Check sheet for the modelled part. Datum: model origin and axes. Units: mm. A direction names the side the tool comes from. Round coordinates to 2 decimals unless told otherwise and drop trailing zeros. Write each loop counter-clockwise with the first axis right and the second up, starting at its lowest first coordinate (ties: lowest second). Pieces come first, ordered by that corner, then holes. Notation, with made-up numbers: (-20.5, 78) -> (-9.5, 78) arc R14 ccw to (-9.5, 95) -> close; hole circle Ø10 at (81, 33). An arc over 180 degrees is marked (long way). One line per item, written item: value.
from build123d import *

# Parameters (mm, degrees)
SKETCH_W     = 40
SKETCH_H     = 7
SKETCH_R     = 1.6
PAD_DEPTH    = 7.25
POCKET_DEPTH = 3
FILLET_R     = 3


with BuildPart() as part:
    # Sketch → Pad (new body)
    with BuildSketch(Plane.XY):
        Rectangle(SKETCH_W, SKETCH_H)
        with Locations((-14.85, 0)):
            Circle(SKETCH_R, mode=Mode.SUBTRACT)
        with Locations((14.85, 0)):
            Circle(SKETCH_R, mode=Mode.SUBTRACT)
    extrude(amount=PAD_DEPTH)

    # Sketch001 (on Face8 of Pad) → Pocket (cut)
    with BuildSketch(Plane.XY.offset(7.25)):
        Polygon((-11.616838, 0), (-13.233419, 2.8), (-16.466581, 2.8), (-18.083162, 0), (-16.466581, -2.8), (-13.233419, -2.8), align=None)
        Polygon((11.616838, 0), (13.233419, -2.8), (16.466581, -2.8), (18.083162, 0), (16.466581, 2.8), (13.233419, 2.8), align=None)
    extrude(amount=-POCKET_DEPTH, mode=Mode.SUBTRACT)

    # Fillet
    fillet_edges = [part.edges().sort_by_distance(p)[0] for p in [
        (20, -3.5, 3.625),
        (20, 3.5, 3.625),
        (-20, 3.5, 3.625),
        (-20, -3.5, 3.625),
    ]]
    fillet(fillet_edges, radius=FILLET_R)


solid = part.part
Item 1: Sectioned sample at D-D (z = 6). Enter the section's corners in (x, y), then the cut area to 3 significant figures.
Result set:
outline: (-20, -0.5) arc R3 ccw to (-17, -3.5) -> (17, -3.5) arc R3 ccw to (20, -0.5) -> (20, 0.5) arc R3 ccw to (17, 3.5) -> (-17, 3.5) arc R3 ccw to (-20, 0.5) -> close; hole (-18.08, 0) -> (-16.47, -2.8) -> (-13.23, -2.8) -> (-11.62, 0) -> (-13.23, 2.8) -> (-16.47, 2.8) -> close; hole (11.62, 0) -> (13.23, -2.8) -> (16.47, -2.8) -> (18.08, 0) -> (16.47, 2.8) -> (13.23, 2.8) -> close
area: 218 mm^2
Item 2: Depth check by flat-ended pin: pin 1 (3.5 mm diameter, centred on x = 14.85, y = 0, fed in from +Z); pin 2 (1 mm diameter, centred on x = -5, y = -1.5, fed in from -Z). Enter the tip coordinate at first touch or a pass-through.
Result set:
pin 1: z = 4.25
pin 2: z = 0
Item 3: Sectioned sample at C-C (y = -2.25). Enter the section's corners in (x, z), then the cut area to 3 significant figures.
Result set:
outline: (-19.44, 0) -> (19.44, 0) -> (19.44, 7.25) -> (16.78, 7.25) -> (16.78, 4.25) -> (12.92, 4.25) -> (12.92, 7.25) -> (-12.92, 7.25) -> (-12.92, 4.25) -> (-16.78, 4.25) -> (-16.78, 7.25) -> (-19.44, 7.25) -> close
area: 259 mm^2
Item 4: Tool access check on faces 1 (the flat face through (-15, -2.8, 6)), 2 (the cylindrical face through (-19.14, -2.6, 3.68)). Record the directions out of +Z, -Z, +X, -X, +Y, -Y that give a thin tool (end or side, any length) a straight path to the whole face; none if there is none.
Result set:
face 1: +Z
face 2: +Z, -Z, -X, -Y
Item 5: Sectioned sample at B-B (z = 1.25). Enter the section's corners in (x, y).
Result set:
outline: (-20, -0.5) arc R3 ccw to (-17, -3.5) -> (17, -3.5) arc R3 ccw to (20, -0.5) -> (20, 0.5) arc R3 ccw to (17, 3.5) -> (-17, 3.5) arc R3 ccw to (-20, 0.5) -> close; hole circle Ø3.2 at (-14.85, 0); hole circle Ø3.2 at (14.85, 0)
Item 6: Sectioned sample at A-A (x = 14.85). Enter the section's corners in (y, z), then the cut area to 4 significant figures.
Result set:
outline: (-3.5, 0) -> (-1.6, 0) -> (-1.6, 4.25) -> (-2.8, 4.25) -> (-2.8, 7.25) -> (-3.5, 7.25) -> close; (1.6, 0) -> (3.5, 0) -> (3.5, 7.25) -> (2.8, 7.25) -> (2.8, 4.25) -> (1.6, 4.25) -> close
area: 20.35 mm^2
Item 7: Material ranges on line 1 along X through (y, z) = (0, 1.75); line 2 along Y through (x, z) = (-14.85, 2.35); line 3 along X through (y, z) = (2.75, 5.75), recorded low to high.
Result set:
line 1: -20 to -16.45, -13.25 to 13.25, 16.45 to 20
line 2: -3.5 to -1.6, 1.6 to 3.5
line 3: -18.98 to -16.5, -13.2 to 13.2, 16.5 to 18.98
Item 8: Release check for a two-part mould opening along Y. For faces 3 (the flat face through (0, 0, 0)), 4 (the cylindrical face through (19.1, -2.64, 3.68)), 5 (the flat face through (-17.264, 1.42, 5.771)), 6 (the flat face through (17.286, 1.38, 5.771)) record: pulls with the +Y half, pulls with the -Y half, needs draft (parallel to the pull), parting line crosses it, or undercut.
Result set:
face 3: needs draft
face 4: pulls with the -Y half
face 5: undercut
face 6: undercut
